```python
from build123d import *

# Parameters (mm, degrees)
SKETCH_W     = 300
SKETCH_H     = 300
PAD_DEPTH    = 19.05
SKETCH001_W  = 19.05
SKETCH001_H  = 9.525
POCKET_DEPTH = 300.001


with BuildPart() as part:
    # Sketch → Pad (new body)
    with BuildSketch(Plane.XY):
        with Locations((150, 150)):
            Rectangle(SKETCH_W, SKETCH_H)
    extrude(amount=PAD_DEPTH)

    # Sketch001 (on Face2 of Pad) → Pocket (cut, through all)
    with BuildSketch(Plane.YZ.offset(300)):
        with Locations((50, 14.2875)):
            Rectangle(SKETCH001_W, SKETCH001_H)
    extrude(amount=-POCKET_DEPTH, mode=Mode.SUBTRACT)


solid = part.part
```
Source: CAD feature listing. Evaluate the final solid. Frame: model axes, mm. A direction names the side the tool comes from. Coordinates: 2 decimals unless noted, no trailing zeros. Write each loop counter-clockwise with the first axis right and the second up, starting at its lowest first coordinate (ties: lowest second). Pieces come first, ordered by that corner, then holes. Notation, with made-up numbers: (-8, 82) -> (15, 82) arc R23 ccw to (15, 114) -> close; hole circle Ø1 at (-38, 74). An arc over 180 degrees is marked (long way). Return JSON: item names as keys, results as strings. Group by question number.
1) Set-up query: faces 1 (the face through (152, 50, 9.525)), 2 (the face through (0, 148, 9)). Return all of +Z, -Z, +X, -X, +Y, -Y with unobstructed straight access to the full face (end or side cutting, diameter ignored); none if empty.
2) Section query A-A, the plane z = 14.25. Return loops of the section in (x, y) (3 decimals).
3) Mould query, pull axis Y, two halves, no side actions, for faces 3 (the face through (148, 300, 9)), 4 (the face through (152, 59.525, 14)), 5 (the face through (148, 152, 0)). Classes: +Y half, -Y half, draft (parallel to the pull), parting line (faces both ways), or undercut.
4) Contact query for a flat-ended pin moving along its axis: P1, Ø5.5, axis at x = 97.5, y = 54, coming from the +Z side (3 decimals). Output: stop coordinate, or through.
5) Section query B-B, the plane x = 267.5. Return loops of the section in (y, z) (3 decimals).
6) Ray query, line 1 along Y through (x, z) = (60, 13.75) (3 decimals); line 2 along Z through (x, y) = (168, 53.5) (3 decimals). Return the intervals inside material, ascending.
From the geometry:
{
 "1": {"face 1": "+Z, +X, -X", "face 2": "+Z, -Z, -X, +Y, -Y"},
 "2": {"outline": "(0, 0) -> (300, 0) -> (300, 40.475) -> (0, 40.475) -> close; (0, 59.525) -> (300, 59.525) -> (300, 300) -> (0, 300) -> close"},
 "3": {"face 3": "+Y half", "face 4": "undercut", "face 5": "draft"},
 "4": {"P1": "z = 9.525"},
 "5": {"outline": "(0, 0) -> (300, 0) -> (300, 19.05) -> (59.525, 19.05) -> (59.525, 9.525) -> (40.475, 9.525) -> (40.475, 19.05) -> (0, 19.05) -> close"},
 "6": {"line 1": "0 to 40.475, 59.525 to 300", "line 2": "0 to 9.525"}
}
